Source: CAD feature listing. Evaluate the final solid. Frame: model axes, mm. A direction names the side the tool comes from. Give positions to 0.01 mm unless a question says otherwise; leave off trailing zeros.
```python
from build123d import *

# Parameters (mm, degrees)
F3_R = 3


with BuildPart() as f2:
    # F2: sweep along a path in F1
    with BuildLine(Plane.YZ) as f2_path:
        Line((0, 0), (0, 30))
        Line((0, 30), (-38.5672565812, 75.9626665871))
        Line((-38.5672565812, 75.9626665871), (-68.1114891716, 81.1721119171))
    # F0 (on Top) → F2 (sweep)
    with BuildSketch(Plane.XY):
        with BuildLine():
            Line((20, -15), (20, 15))
            Line((20, 15), (10, 15))
            add(Edge.make_bspline(
                [(10, 15), (12.3940897704, 9.9797566054), (16.8411980376, 0.6544730759), (11.1651576872, -12.4181404175), (3.6445260134, -12.6084000337), (0, -12.7006005496)],
                knots=[0, 0, 0, 0, 0.3753981471, 0.6973156246, 1, 1, 1, 1], degree=3))
            add(Edge.make_bspline(
                [(-10, 15), (-12.3940897704, 9.9797566054), (-16.8411980376, 0.6544730759), (-11.1651576872, -12.4181404175), (-3.6445260134, -12.6084000337), (0, -12.7006005496)],
                knots=[0, 0, 0, 0, 0.3753981471, 0.6973156246, 1, 1, 1, 1], degree=3))
            Line((-10, 15), (-20, 15))
            Line((-20, 15), (-20, -15))
            Line((-20, -15), (20, -15))
        make_face()
    sweep(path=f2_path.line, transition=Transition.RIGHT)

    # F3
    f3_edges = [f2.edges().sort_by_distance(p)[0] for p in [
        (-20, 15, 17.729777),
        (-20, -7.792962, 62.623147),
        (-20, -48.046345, 92.865485),
        (-20, -15, 12.270223),
        (-20, -30.774295, 43.339519),
        (-20, -58.632401, 64.269294),
        (20, -48.046345, 92.865485),
        (20, -7.792962, 62.623147),
        (20, 15, 17.729777),
        (20, -15, 12.270223),
        (20, -30.774295, 43.339519),
        (20, -58.632401, 64.269294),
    ]]
    fillet(f3_edges, radius=F3_R)


solid = f2.part
```
(1) Reachability of faces 1 (the cylindrical face through (19.145, -8.803, 62.424)), 2 (the cylindrical face through (-19.14, -14.1, 13)) from +Z, -Z, +X, -X, +Y, -Y: full face, straight path, thin tool, end or side. Return the list, or none.
A:
face 1: +Z, +X, +Y
face 2: -Z, -X, -Y
(2) First-contact query: pin 1 (8 mm diameter, centred on x = -12.5, z = 12, fed in from -Y); pin 2 (12 mm diameter, centred on x = 7, y = -21.5, fed in from -Z); pin 3 (6 mm diameter, centred on x = -10, y = -23, fed in from -Z). Flat tips, straight axial feed; report the tip coordinate or a pass-through.
A:
pin 1: stops at y = -15
pin 2: stops at z = 25.14
pin 3: stops at z = 30.5
(3) Ray query, line 1 along X through (y, z) = (-48.5, 67); line 2 along X through (y, z) = (-22, 69.5); line 3 along Z through (x, y) = (-2, -19). Return the intervals inside material, ascending.
A:
line 1: x = -20 to -10, 10 to 20
line 2: x = -20 to -12.89, 12.89 to 20
line 3: z = 29.31 to 32.98
